```python
from build123d import *
from OCP.BRepFilletAPI import BRepFilletAPI_MakeChamfer

# Parameters (mm, degrees)
SKETCH_2_R          = 0.825
SKETCH_2_R_2        = 6
EXTRUDE_1_DEPTH     = 2
SKETCH_4_R          = 1.6
CUT_EXTRUDE_1_DEPTH = 15
EXTRUDE_2_DEPTH     = 2
EXTRUDE_3_DEPTH     = 2
CHAMFER_2_SIZE      = 20
SKETCH_8_W          = 95
SKETCH_8_H          = 22
EXTRUDE_4_DEPTH     = 2
CHAMFER_3_SIZE      = 12
CHAMFER_4_SIZE      = 10
CHAMFER_4_SIZE2     = 7.162801166
SKETCH_10_R         = 1.65
CUT_EXTRUDE_2_DEPTH = 14


with BuildPart() as part:
    # 草图2 → 凸台-拉伸1 (new, symmetric)
    with BuildSketch(Plane.XY):
        Polygon((10.355339059, 25), (-10.355339059, 25), (-25, 10.355339059), (-25, -10.355339059), (-10.355339059, -25), (10.355339059, -25), (25, -10.355339059), (25, 10.355339059), align=None)
        with Locations((-16.5, 0)):
            Circle(SKETCH_2_R, mode=Mode.SUBTRACT)
        with Locations((0, 16.5)):
            Circle(SKETCH_2_R, mode=Mode.SUBTRACT)
        with Locations((16.5, 0)):
            Circle(SKETCH_2_R, mode=Mode.SUBTRACT)
        with Locations((0, -16.5)):
            Circle(SKETCH_2_R, mode=Mode.SUBTRACT)
        Circle(SKETCH_2_R_2, mode=Mode.SUBTRACT)
    extrude(amount=EXTRUDE_1_DEPTH, both=True)

    # 草图4 → 切除-拉伸1 (cut)
    with BuildSketch(Plane(origin=(0, 0, -2), x_dir=(-1, 0, 0), z_dir=(0, 0, -1))):
        with Locations((-7.5, -20)):
            Circle(SKETCH_4_R)
        with Locations(Location((7.5, -20, 0), (0, 0, 180))):
            Circle(SKETCH_4_R)
        with Locations((-20, 7.5)):
            Circle(SKETCH_4_R)
        with Locations(Location((-20, -7.5, 0), (0, 0, 180))):
            Circle(SKETCH_4_R)
        with Locations((7.5, 20)):
            Circle(SKETCH_4_R)
        with Locations(Location((-7.5, 20, 0), (0, 0, 180))):
            Circle(SKETCH_4_R)
        with Locations((20, -7.5)):
            Circle(SKETCH_4_R)
        with Locations(Location((20, 7.5, 0), (0, 0, 180))):
            Circle(SKETCH_4_R)
    extrude(amount=-CUT_EXTRUDE_1_DEPTH, mode=Mode.SUBTRACT)

    # 草图5 → 凸台-拉伸2 (add, symmetric)
    with BuildSketch(Plane.XY):
        Polygon((-25, -10.355339059), (-92.5, -73), (-70, -73), (-16.17766953, -19.17766953), align=None)
        Polygon((70, -73), (92.5, -73), (25, -10.355339059), (16.17766953, -19.17766953), align=None)
    extrude(amount=EXTRUDE_2_DEPTH, both=True)

    # 草图6 → 凸台-拉伸3 (add, symmetric)
    with BuildSketch(Plane.XY):
        Polygon((-70, -73), (-45, -73), (-10.355339059, -25), (-16.17766953, -19.17766953), align=None)
        Polygon((70, -73), (16.17766953, -19.17766953), (10.355339059, -25), (45, -73), align=None)
    extrude(amount=EXTRUDE_3_DEPTH, both=True)

    # 倒角2
    chamfer_2_edges = [part.edges().sort_by_distance(p)[0] for p in [
        (-92.5, -73, 0),
        (92.5, -73, 0),
    ]]
    chamfer(chamfer_2_edges, length=CHAMFER_2_SIZE)

    # 草图8 → 凸台-拉伸4 (add, symmetric)
    with BuildSketch(Plane.XY):
        with Locations((0, -70)):
            Rectangle(SKETCH_8_W, SKETCH_8_H)
    extrude(amount=EXTRUDE_4_DEPTH, both=True)

    # 倒角3
    # the kernel refuses this chamfer: 12 mm, written as the material it takes off along each edge
    with BuildSketch(Plane(origin=(47.5, -81, -32.860195856), x_dir=(0.02749587661058619, 0.9996219169112968, 0), z_dir=(0, 0, 1))) as chamfer_3_piece_1_section:
        Polygon((CHAMFER_3_SIZE * 0.999621916911, CHAMFER_3_SIZE * 0.0274958766106), (-CHAMFER_3_SIZE * 0.0274958766106, CHAMFER_3_SIZE * 0.999621916911), (0, 0), align=None)
    chamfer_3_piece_1 = extrude(amount=65.720391711, mode=Mode.PRIVATE)
    chamfer_3_piece_1 = split(chamfer_3_piece_1, bisect_by=Plane(origin=(43.13163598, -73, 0), z_dir=(0, -1, 0)), keep=Keep.TOP, mode=Mode.PRIVATE)
    add(chamfer_3_piece_1, mode=Mode.SUBTRACT)
    with BuildSketch(Plane(origin=(-47.5, -81, 32.860195856), x_dir=(-0.02749587661058619, 0.9996219169112968, 0), z_dir=(0, 0, -1))) as chamfer_3_piece_2_section:
        Polygon((CHAMFER_3_SIZE * 0.999621916911, CHAMFER_3_SIZE * 0.0274958766106), (-CHAMFER_3_SIZE * 0.0274958766106, CHAMFER_3_SIZE * 0.999621916911), (0, 0), align=None)
    chamfer_3_piece_2 = extrude(amount=65.720391711, mode=Mode.PRIVATE)
    chamfer_3_piece_2 = split(chamfer_3_piece_2, bisect_by=Plane(origin=(-43.13163598, -73, 0), z_dir=(0, -1, 0)), keep=Keep.TOP, mode=Mode.PRIVATE)
    add(chamfer_3_piece_2, mode=Mode.SUBTRACT)

    # 倒角4: one chamfer whose edges measure the first distance from different faces: ONE call of the kernel's chamfer builder (chamfer() names one face for all edges)
    chamfer_4_edges_1 = [part.edges().sort_by_distance(p)[0] for p in [
        (34.895307226, -59, 0),
    ]]
    chamfer_4_side_1 = [part.faces().sort_by_distance(p)[0] for p in [
        (22.625323142, -42, 0),
    ]]
    chamfer_4_edges_2 = [part.edges().sort_by_distance(p)[0] for p in [
        (-34.895307226, -59, 0),
    ]]
    chamfer_4_side_2 = [part.faces().sort_by_distance(p)[0] for p in [
        (-22.625323142, -42, 0),
    ]]
    chamfer_4 = BRepFilletAPI_MakeChamfer(part.part.solid().wrapped)
    for e in chamfer_4_edges_1:
        chamfer_4.Add(CHAMFER_4_SIZE, CHAMFER_4_SIZE2, e.wrapped, chamfer_4_side_1[0].wrapped)  # the first distance lies on this face
    for e in chamfer_4_edges_2:
        chamfer_4.Add(CHAMFER_4_SIZE, CHAMFER_4_SIZE2, e.wrapped, chamfer_4_side_2[0].wrapped)  # the first distance lies on this face
    add(Compound.cast(chamfer_4.Shape()), mode=Mode.REPLACE)

    # 草图10 → 切除-拉伸2 (cut)
    with BuildSketch(Plane.XY.offset(2)):
        with Locations((-17.5, -76)):
            Circle(SKETCH_10_R)
        with Locations((17.5, -76)):
            Circle(SKETCH_10_R)
    extrude(amount=-CUT_EXTRUDE_2_DEPTH, mode=Mode.SUBTRACT)


solid = part.part
```
Geometry: final body of the model. Coordinates: model frame, mm. A direction names the side the tool comes from. Coordinates: 2 decimals unless noted, no trailing zeros. Order: outer loops, then holes, each group sorted by start corner. A loop starts at its lowest first (then second) coordinate and runs counter-clockwise, first axis right, second up. Notation, with made-up numbers: (-19.75, -38) - (-6.75, -38) arc R32 cw to (-6.75, -2) - close; hole circle Ø9 at (44.25, 11.25). An arc over 180 degrees is marked (long way). Write each question's results on one line, items separated by ' | '.
(1) Line query: line 1 (Y direction, x = -7.5, z = -0.3); line 2 (Y direction, x = -9.5, z = 1.75); line 3 (Y direction, x = 2.5, z = -1.5). Output: solid intervals per line, ascending. Write a range as [from, to].
Values found:
line 1: y = [-81, -59], [-25, -21.6], [-18.4, 18.4], [21.6, 25] | line 2: y = [-81, -59], [-25, 25] | line 3: y = [-81, -59], [-25, -5.45], [5.45, 25]
(2) Set-up query: faces 1 (the face through (39.6, -76.9, 0)), 2 (the face through (0, -59, 0)). Return all of +Z, -Z, +X, -X, +Y, -Y with unobstructed straight access to the full face (end or side cutting, diameter ignored); none if empty.
Values found:
face 1: +Z, -Z, +X, -Y | face 2: +Z, -Z
(3) Mould query, pull axis Y, two halves, no side actions, for faces 3 (the face through (-58, -73, 0)), 4 (the face through (16, -27, -2)), 5 (the face through (-7.292, 21.586, -0.028)). Classes: +Y half, -Y half, draft (parallel to the pull), parting line (faces both ways), or undercut.
Values found:
face 3: -Y half | face 4: draft | face 5: undercut
(4) Section query C-C, the plane y = -35. Return the cut outline in (x, z).
Values found:
outline: (-51.55, -2) - (-17.57, -2) - (-17.57, 2) - (-51.55, 2) - close; (17.57, -2) - (51.55, -2) - (51.55, 2) - (17.57, 2) - close
(5) First-contact query: pin 1 Ø2 at (x, z) = (63.5, 0.5) entering from -Y; pin 2 Ø1 at (y, z) = (12, 1) entering from -X. Flat tips, straight axial feed; report the tip coordinate or a pass-through.
Values found:
pin 1: stops at y = -73 | pin 2: stops at x = -23.86
(6) Section query B-B, the plane x = -14. Return the cut outline in (y, z).
Values found:
outline: (-81, -2) - (-59, -2) - (-59, 2) - (-81, 2) - close; (-30.05, -2) - (21.36, -2) - (21.36, 2) - (-30.05, 2) - close
(7) Section query D-D, the plane z = 0.1. Count the separate pieces of the cut face and the enclosed holes in it, plus the area to 3 significant figures.
Values found:
separate pieces: 1 | enclosed holes: 16 | area: 7,590 mm²
(8) Section query A-A, the plane y = -20. Return the cut outline in (x, z).
Values found:
outline: (-35.39, -2) - (-9.1, -2) - (-9.1, 2) - (-35.39, 2) - close; (-5.9, -2) - (5.9, -2) - (5.9, 2) - (-5.9, 2) - close; (9.1, -2) - (35.39, -2) - (35.39, 2) - (9.1, 2) - close
